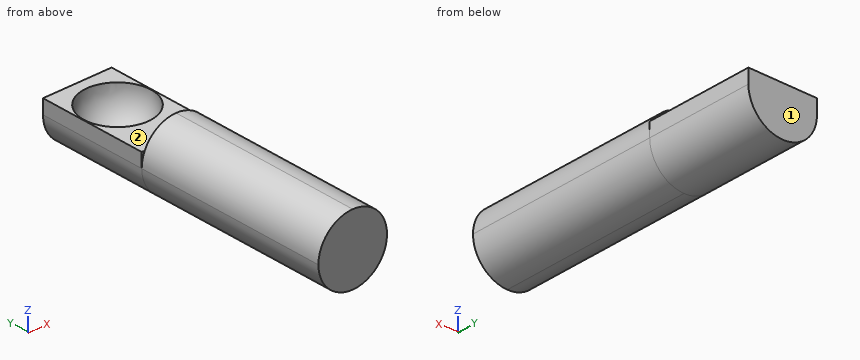
from build123d import *

# Parameters (mm, degrees)
SKETCH1_W           = 5.1
SKETCH1_H           = 22.6
BOSS_EXTRUDE1_DEPTH = 2.55
SKETCH3_W           = 5.1
SKETCH3_H           = 8.1
BOSS_EXTRUDE2_DEPTH = 1
CUT_EXTRUDE1_DEPTH  = 14.5
SKETCH5_W           = 5.1
SKETCH5_H           = 1.5
CUT_EXTRUDE2_DEPTH  = 8.1
CUT_EXTRUDE3_DEPTH  = 16.144470938


with BuildPart() as part:
    # Sketch1 → Boss-Extrude1 (new, symmetric)
    with BuildSketch(Plane.XY):
        Rectangle(SKETCH1_W, SKETCH1_H)
    extrude(amount=BOSS_EXTRUDE1_DEPTH, both=True)

    # Sketch3 → Boss-Extrude2 (add)
    with BuildSketch(Plane(origin=(0, 0, -2.55), x_dir=(-1, 0, 0), z_dir=(0, 0, -1))):
        with Locations((0, 7.25)):
            Rectangle(SKETCH3_W, SKETCH3_H)
    extrude(amount=BOSS_EXTRUDE2_DEPTH)

    # Sketch4 → Cut-Extrude1 (cut)
    with BuildSketch(Plane.XZ.offset(11.3)):
        with BuildLine():
            Line((0, 2.55), (-2.55, 2.55))
            Line((-2.55, 2.55), (-2.55, 0))
            ThreePointArc((-2.55, 0), (-1.803122292, 1.803122292), (0, 2.55))
        make_face()
        with BuildLine():
            Line((2.55, 2.55), (0, 2.55))
            ThreePointArc((0, 2.55), (1.803122292, 1.803122292), (2.55, 0))
            Line((2.55, 0), (2.55, 2.55))
        make_face()
        with BuildLine():
            ThreePointArc((2.55, 0), (1.803122292, -1.803122292), (0, -2.55))
            Line((0, -2.55), (2.55, -2.55))
            Line((2.55, -2.55), (2.55, 0))
        make_face()
        with BuildLine():
            ThreePointArc((0, -2.55), (-1.803122292, -1.803122292), (-2.55, 0))
            Line((-2.55, 0), (-2.55, -2.55))
            Line((-2.55, -2.55), (0, -2.55))
        make_face()
    extrude(amount=-CUT_EXTRUDE1_DEPTH, mode=Mode.SUBTRACT)

    # Sketch5 → Cut-Extrude2 (cut)
    with BuildSketch(Plane(origin=(0, 11.3, 0), x_dir=(1, 0, 0), z_dir=(0, 1, 0))):
        with Locations((0, -1.8)):
            Rectangle(SKETCH5_W, SKETCH5_H)
    extrude(amount=-CUT_EXTRUDE2_DEPTH, mode=Mode.SUBTRACT)

    # Sketch6 → Cut-Revolve2 (revolve, cut)
    with BuildSketch(Plane.XY.offset(1.05)):
        with BuildLine():
            Line((-2.5, 8), (2.5, 8))
            ThreePointArc((2.5, 8), (0, 5.5), (-2.5, 8))
        make_face()
    revolve(axis=Axis((-2.5, 8, 1.05), (1, 0, 0)), mode=Mode.SUBTRACT)

    # Sketch7 → Cut-Extrude3 (cut, through all)
    with BuildSketch(Plane.XZ.offset(-3.2)):
        with BuildLine():
            Line((-2.55, -3.55), (2.55, -3.55))
            Line((2.55, -3.55), (2.55, 0))
            ThreePointArc((2.55, 0), (0, -2.55), (-2.55, 0))
            Line((-2.55, 0), (-2.55, -3.55))
        make_face()
    extrude(amount=-CUT_EXTRUDE3_DEPTH, mode=Mode.SUBTRACT)


solid = part.part
Source: CAD feature listing. Evaluate the final solid. Frame: model axes, mm. Face numbers are marked on the shaded views. A direction names the side the tool comes from. Coordinates: 2 decimals unless noted, no trailing zeros. Loops run counter-clockwise (first coordinate to the right, second up) from the corner with the lowest first, then second, coordinate; pieces in that order, holes last. Notation, with made-up numbers: (-25.75, -29.75) -> (-19.75, -29.75) arc R27 cw to (-19.75, 3.25) -> close; hole circle Ø9 at (12.5, -14.5). An arc over 180 degrees is marked (long way). Answer in a Markdown table with one row per item. Add a question column.
Q1. Section B-B on y = 0. Return the cut outline in (x, z), and give its area (3 significant figures).
Q2. Contact query for flat-ended pins moving along their axis: pin 1 Ø2 at (x, y) = (-1.5, 7) entering from +Z; pin 2 Ø1.2 at (x, z) = (1, 2) entering from +Y. Output: stop coordinate, or through.
Q3. Ray query, line 1 along Y through (x, z) = (1.35, 2); line 2 along Y through (x, z) = (-0.2, -1.2); line 3 along Y through (x, z) = (0.4, 0.45). Return the intervals inside material, ascending.
Q4. Reachability of the marked faces 1 and 2 from +Z, -Z, +X, -X, +Y, -Y: full face, straight path, thin tool, end or side. Return the list, or none.
Q5. Section D-D on z = -2.15. Return the cut outline in (x, y).
Q6. Section A-A on z = -0.2. Return the cut outline in (x, y).
Q7. Section C-C on x = 1.6. Return the cut outline in (y, z).
Computed values:
| question | item | result |
|---|---|---|
| 1 | outline | circle Ø5.1 at (0, 0) |
| 1 | area | 20.4 mm^2 |
| 2 | pin 1 | stops at z = 1.05 |
| 2 | pin 2 | stops at y = 3.2 |
| 3 | line 1 | y = -11.3 to 3.2 |
| 3 | line 2 | y = -11.3 to 6.93, 9.07 to 11.3 |
| 3 | line 3 | y = -11.3 to 5.61, 10.39 to 11.3 |
| 4 | face 1 | +Z, -Z, +X, -X, +Y |
| 4 | face 2 | +Z, +X, -X, +Y |
| 5 | outline | (-1.37, -11.3) -> (1.37, -11.3) -> (1.37, 11.3) -> (-1.37, 11.3) -> close |
| 6 | outline | (-2.54, -11.3) -> (2.54, -11.3) -> (2.54, 11.3) -> (-2.54, 11.3) -> close; hole circle Ø4.33 at (0, 8) |
| 7 | outline | (-11.3, -1.99) -> (11.3, -1.99) -> (11.3, 1.05) -> (9.92, 1.05) arc R1.92 cw to (6.08, 1.05) -> (3.2, 1.05) -> (3.2, 1.99) -> (-11.3, 1.99) -> close |
